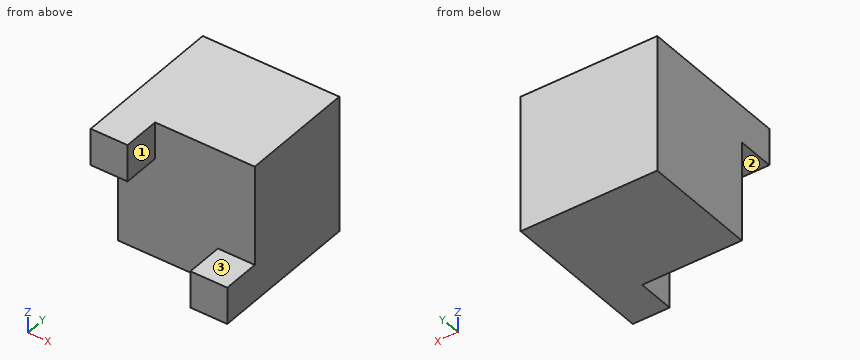
```python
from build123d import *

# Parameters (mm, degrees)
F0_W       = 50.8
F0_H       = 50.8
F1_DEPTH   = 24.892
F2_W       = 13.716
F2_H       = 13.716
F3_DEPTH   = 13.97
F5_W       = 50.8
F5_H       = 50.8
F1_FACE1_W = 50.8
F1_FACE1_H = 50.8
F6_DEPTH   = 18.034


with BuildPart() as f1:
    # F0 (on Front) → F1 (new body)
    with BuildSketch(Plane.XZ):
        with Locations((-25.4, 25.4)):
            Rectangle(F0_W, F0_H)
    extrude(amount=-F1_DEPTH)

    # F2 (on face) → F3 (join)
    with BuildSketch(Plane.XZ):
        with Locations((-43.942, 43.942)):
            Rectangle(F2_W, F2_H)
        with Locations((-6.858, 6.858)):
            Rectangle(F2_W, F2_H)
    extrude(amount=F3_DEPTH)

    # F5 (on face) + F4 (on face) + F1_face1 (on face) → F6 (join, symmetric)
    with BuildSketch(Plane(origin=(0, 24.892, 0), x_dir=(-1, 0, 0), z_dir=(0, 1, 0))):
        with Locations((25.4, 25.4)):
            Rectangle(F5_W, F5_H)
    with BuildSketch(Plane(origin=(0, 24.892, 0), x_dir=(-1, 0, 0), z_dir=(0, 1, 0))):
        Polygon((13.716, 0), (37.084, 0), (37.084, 13.5469082743), (50.8, 13.5469082743), (50.8, 36.3148450851), (37.084, 36.3148450851), (37.084, 50.8), (13.716, 50.8), (13.716, 35.1472571492), (0, 35.1472571492), (0, 12.9631143063), (13.716, 12.9631143063), align=None)
    with BuildSketch(Plane(origin=(-25.4, 24.892, 25.4), x_dir=(1, 0, 0), z_dir=(0, 1, 0))):
        Rectangle(F1_FACE1_W, F1_FACE1_H)
    extrude(amount=F6_DEPTH, both=True)


solid = f1.part
```
Could you check a few things on this model? Use its own coordinates, in mm. Face numbers are marked on the shaded views. A direction names the side the tool comes from. Give positions to 0.01 mm unless a question says otherwise; leave off trailing zeros. Write each loop counter-clockwise with the first axis right and the second up, starting at its lowest first coordinate (ties: lowest second). Pieces come first, ordered by that corner, then holes. Notation, with made-up numbers: (-2, 85.5) - (17, 85.5) arc R12 ccw to (17, 105.5) - close; hole circle Ø7 at (67, 43.25). An arc over 180 degrees is marked (long way). One line per item, written item: value. Start each with the question number.
Item 1: I'm going to push flat-ended pins straight in: pin 1 (4 mm diameter, centred on y = -3.5, z = 8, fed in from -X); pin 2 (1 mm diameter, centred on x = -22.5, z = 31, fed in from -Y); pin 3 (11 mm diameter, centred on x = -43, y = -8.5, fed in from -Z); pin 4 (2 mm diameter, centred on y = 32, z = 42, fed in from +X). Where does each tip first touch, or does it pass through?
Item 2: Which directions (+Z, -Z, +X, -X, +Y, -Y) give clear straight access to the entire face, cutting with the end or side of a thin tool? Please do the marked faces 1, 2 and 3.
Item 3: Imagine slicing it at C-C, the plane z = 40. List the corners of the cut face in (x, y) for me, and give its area (3 significant figures).
Item 4: Please list where these lines run through material, in increasing order: line 1 (Y direction, x = -36, z = 23); line 2 (X direction, y = -1, z = 46); line 3 (X direction, y = -8, z = 13.5). Write a range as from..to.
Item 5: Imagine slicing it at B-B, the plane x = -47.5. List the corners of the cut face in (y, z) for me, and give its area (3 significant figures).
Item 6: Imagine slicing it at A-A, the plane y = -5.5. List the corners of the cut face in (x, z) for me, and give its area (3 significant figures).
Item 7: Imagine slicing it at D-D, the plane x = -25. List the corners of the cut face in (y, z) for me, and give its area (3 significant figures).
Geometry says:
1. pin 1: x = -13.72
1. pin 2: y = 0
1. pin 3: z = 37.08
1. pin 4: x = 0
2. face 1: +Z, -Z, +X, -Y
2. face 2: -Z, +X, -X, -Y
2. face 3: +Z, +X, -X, -Y
3. outline: (-50.8, -13.97) - (-37.08, -13.97) - (-37.08, 0) - (0, 0) - (0, 42.93) - (-50.8, 42.93) - close
3. area: 2,370 mm^2
4. line 1: 0..42.93
4. line 2: -50.8..-37.08
4. line 3: -13.72..0
5. outline: (-13.97, 37.08) - (0, 37.08) - (0, 0) - (42.93, 0) - (42.93, 50.8) - (-13.97, 50.8) - close
5. area: 2,370 mm^2
6. outline: (-50.8, 37.08) - (-37.08, 37.08) - (-37.08, 50.8) - (-50.8, 50.8) - close; (-13.72, 0) - (0, 0) - (0, 13.72) - (-13.72, 13.72) - close
6. area: 376 mm^2
7. outline: (0, 0) - (42.93, 0) - (42.93, 50.8) - (0, 50.8) - close
7. area: 2,180 mm^2
